from build123d import *

# Parameters (mm, degrees)
F0_W     = 32
F0_H     = 32
F1_DEPTH = 160
F2_T     = -2
F4_DEPTH = 2


with BuildPart() as f1:
    # F0 (on Front) → F1 (new body)
    with BuildSketch(Plane.XZ):
        with Locations((16, 16)):
            Rectangle(F0_W, F0_H)
    extrude(amount=-F1_DEPTH)

    # F2
    f2_openings = [f1.faces().sort_by_distance(p)[0] for p in [
        (16, 0, 16),
        (0, 80, 16),
        (16, 160, 16),
    ]]
    offset(amount=F2_T, openings=f2_openings)

    # F3 (on face) → F4 (cut, through all)
    with BuildSketch(Plane.XY.offset(32)):
        with BuildLine():
            Line((16, 25.999), (16, 23.999))
            Line((16, 23.999), (17.847759065, 23.2336331353))
            ThreePointArc((17.847759065, 23.2336331353), (17.9615705608, 23.608819356), (18, 23.999))
            ThreePointArc((18, 23.999), (17.4142135624, 25.4132135624), (16, 25.999))
        make_face()
        with BuildLine():
            ThreePointArc((16, 25.999), (14.3370607754, 25.110140466), (14.152240935, 23.2336331353))
            Line((14.152240935, 23.2336331353), (16, 23.999))
            Line((16, 23.999), (16, 25.999))
        make_face()
        with BuildLine():
            ThreePointArc((14.152240935, 23.2336331353), (14.888859534, 22.3360607754), (16, 21.999))
            Line((16, 21.999), (16, 23.999))
            Line((16, 23.999), (14.152240935, 23.2336331353))
        make_face()
        with BuildLine():
            Line((16, 23.999), (16, 21.999))
            ThreePointArc((16, 21.999), (17.111140466, 22.3360607754), (17.847759065, 23.2336331353))
            Line((17.847759065, 23.2336331353), (16, 23.999))
        make_face()
        with BuildLine():
            Line((14.152240935, 8.7643668647), (16, 7.999))
            Line((16, 7.999), (16, 9.999))
            ThreePointArc((16, 9.999), (14.888859534, 9.6619392246), (14.152240935, 8.7643668647))
        make_face()
        with BuildLine():
            Line((16, 9.999), (16, 7.999))
            Line((16, 7.999), (17.847759065, 8.7643668647))
            ThreePointArc((17.847759065, 8.7643668647), (17.111140466, 9.6619392246), (16, 9.999))
        make_face()
        with BuildLine():
            Line((16, 7.999), (16, 5.999))
            ThreePointArc((16, 5.999), (17.4142135624, 6.5847864376), (18, 7.999))
            ThreePointArc((18, 7.999), (17.9615705608, 8.389180644), (17.847759065, 8.7643668647))
            Line((17.847759065, 8.7643668647), (16, 7.999))
        make_face()
        with BuildLine():
            ThreePointArc((14.152240935, 8.7643668647), (14.3370607754, 6.887859534), (16, 5.999))
            Line((16, 5.999), (16, 7.999))
            Line((16, 7.999), (14.152240935, 8.7643668647))
        make_face()
        with BuildLine():
            ThreePointArc((18, 39.999), (17.4142135624, 41.4132135624), (16, 41.999))
            Line((16, 41.999), (16, 39.999))
            Line((16, 39.999), (16, 37.999))
            ThreePointArc((16, 37.999), (17.4142135624, 38.5847864376), (18, 39.999))
        make_face()
        with BuildLine():
            Line((16, 39.999), (16, 41.999))
            ThreePointArc((16, 41.999), (14, 39.999), (16, 37.999))
            Line((16, 37.999), (16, 39.999))
        make_face()
        with BuildLine():
            Line((16, 55.999), (16, 57.999))
            ThreePointArc((16, 57.999), (14, 55.999), (16, 53.999))
            Line((16, 53.999), (16, 55.999))
        make_face()
        with BuildLine():
            ThreePointArc((18, 55.999), (17.4142135624, 57.4132135624), (16, 57.999))
            Line((16, 57.999), (16, 55.999))
            Line((16, 55.999), (16, 53.999))
            ThreePointArc((16, 53.999), (17.4142135624, 54.5847864376), (18, 55.999))
        make_face()
        with BuildLine():
            Line((16, 71.999), (16, 73.999))
            ThreePointArc((16, 73.999), (14, 71.999), (16, 69.999))
            Line((16, 69.999), (16, 71.999))
        make_face()
        with BuildLine():
            ThreePointArc((18, 71.999), (17.4142135624, 73.4132135624), (16, 73.999))
            Line((16, 73.999), (16, 71.999))
            Line((16, 71.999), (16, 69.999))
            ThreePointArc((16, 69.999), (17.4142135624, 70.5847864376), (18, 71.999))
        make_face()
        with BuildLine():
            ThreePointArc((16, 90.001), (14, 88.001), (16, 86.001))
            Line((16, 86.001), (16, 90.001))
        make_face()
        with BuildLine():
            Line((16, 90.001), (16, 86.001))
            ThreePointArc((16, 86.001), (17.4142135624, 86.5867864376), (18, 88.001))
            ThreePointArc((18, 88.001), (17.4142135624, 89.4152135624), (16, 90.001))
        make_face()
        with BuildLine():
            Line((16, 106.001), (16, 102.001))
            ThreePointArc((16, 102.001), (17.4142135624, 102.5867864376), (18, 104.001))
            ThreePointArc((18, 104.001), (17.4142135624, 105.4152135624), (16, 106.001))
        make_face()
        with BuildLine():
            ThreePointArc((16, 106.001), (14, 104.001), (16, 102.001))
            Line((16, 102.001), (16, 106.001))
        make_face()
        with BuildLine():
            ThreePointArc((16, 122.001), (14, 120.001), (16, 118.001))
            Line((16, 118.001), (16, 122.001))
        make_face()
        with BuildLine():
            Line((16, 122.001), (16, 118.001))
            ThreePointArc((16, 118.001), (17.4142135624, 118.5867864376), (18, 120.001))
            ThreePointArc((18, 120.001), (17.4142135624, 121.4152135624), (16, 122.001))
        make_face()
        with BuildLine():
            Line((16, 134.001), (16, 138.001))
            ThreePointArc((16, 138.001), (14, 136.001), (16, 134.001))
        make_face()
        with BuildLine():
            ThreePointArc((18, 136.001), (17.4142135624, 137.4152135624), (16, 138.001))
            Line((16, 138.001), (16, 134.001))
            ThreePointArc((16, 134.001), (17.4142135624, 134.5867864376), (18, 136.001))
        make_face()
        with BuildLine():
            Line((16, 150.001), (16, 154.001))
            ThreePointArc((16, 154.001), (14, 152.001), (16, 150.001))
        make_face()
        with BuildLine():
            ThreePointArc((18, 152.001), (17.4142135624, 153.4152135624), (16, 154.001))
            Line((16, 154.001), (16, 150.001))
            ThreePointArc((16, 150.001), (17.4142135624, 150.5867864376), (18, 152.001))
        make_face()
        with BuildLine():
            ThreePointArc((16, 20.19), (11.809, 15.999), (16, 11.808))
            Line((16, 11.808), (16, 20.19))
        make_face()
        with BuildLine():
            Line((16, 20.19), (16, 11.808))
            ThreePointArc((16, 11.808), (18.96348452, 13.03551548), (20.191, 15.999))
            ThreePointArc((20.191, 15.999), (18.96348452, 18.96248452), (16, 20.19))
        make_face()
        with BuildLine():
            Line((16, 139.81), (16, 148.192))
            ThreePointArc((16, 148.192), (11.809, 144.001), (16, 139.81))
        make_face()
        with BuildLine():
            ThreePointArc((20.191, 144.001), (18.96348452, 146.96448452), (16, 148.192))
            Line((16, 148.192), (16, 139.81))
            ThreePointArc((16, 139.81), (18.96348452, 141.03751548), (20.191, 144.001))
        make_face()
    extrude(amount=-F4_DEPTH, mode=Mode.SUBTRACT)


solid = f1.part
Part model, mm, in its own coordinate system. A direction names the side the tool comes from. Give positions to 0.01 mm unless a question says otherwise; leave off trailing zeros. Order: outer loops, then holes, each group sorted by start corner. A loop starts at its lowest first (then second) coordinate and runs counter-clockwise, first axis right, second up. Notation, with made-up numbers: (9, 2) -> (41, 2) arc R17 ccw to (41, 32) -> close; hole circle Ø1 at (53, 50.5). An arc over 180 degrees is marked (long way). Use one line per item in the form item = value.
(1) Saw through at A-A (x = 5). Write the cut outline in (y, z).
Solution:
outline = (0, 0) -> (160, 0) -> (160, 2) -> (0, 2) -> close; (0, 30) -> (160, 30) -> (160, 32) -> (0, 32) -> close
(2) Saw through at B-B (y = 110.5). Write the cut outline in (x, z), then the cut area to 3 significant figures.
Solution:
outline = (0, 0) -> (32, 0) -> (32, 32) -> (0, 32) -> (0, 30) -> (30, 30) -> (30, 2) -> (0, 2) -> close
area = 184 mm²
(3) Saw through at C-C (z = 6.5). Write the cut outline in (x, y).
Solution:
outline = (30, 0) -> (32, 0) -> (32, 160) -> (30, 160) -> close
(4) Flat gauge pin, fed straight in: P1, Ø8, axis at x = 7, y = 88, coming from the -Z side. Where does the tip first touch, or does it go through?
Solution:
P1 = 0
(5) Tool access for faces 4 (the face through (31, 0, 15)), 5 (the face through (15, 79, 2)): list every direction of +Z, -Z, +X, -X, +Y, -Y with a clear straight run to the whole face (end or side of a thin tool).
Solution:
face_4 = +Z, -Z, +X, -X, -Y
face_5 = -X, +Y, -Y
(6) Pull direction Z, two halves, no side cores. Call faces 1 (the face through (30, 79, 16)), 2 (the face through (16, 79, 0)), 3 (the face through (32, 79, 16)): +Z half, -Z half, draft (parallel to the pull), parting line (faces both ways), or undercut.
Solution:
face_1 = undercut
face_2 = -Z half
face_3 = draft
(7) Drill centre lines: line 1 (Z direction, x = 12, y = 116.5); line 2 (X direction, y = 80.5, z = 24); line 3 (Z direction, x = 16, y = 86.5). Where is each one in solid material? Low to high. Write a range as from..to.
Solution:
line_1 = 0..2, 30..32
line_2 = 30..32
line_3 = 0..2
